Drawing for the job (mm, zero at the part's lowest x, y, z). Round coordinates to 2 decimals unless told otherwise and drop trailing zeros. Loops run counter-clockwise (first coordinate to the right, second up) from the corner with the lowest first, then second, coordinate; pieces in that order, holes last. Notation, with made-up numbers: (47, 3.5) - (86, 3.5) arc R10 ccw to (86, 8.5) - close; hole circle Ø1 at (-3, 57). An arc over 180 degrees is marked (long way). Put each result on its own line as item: value.
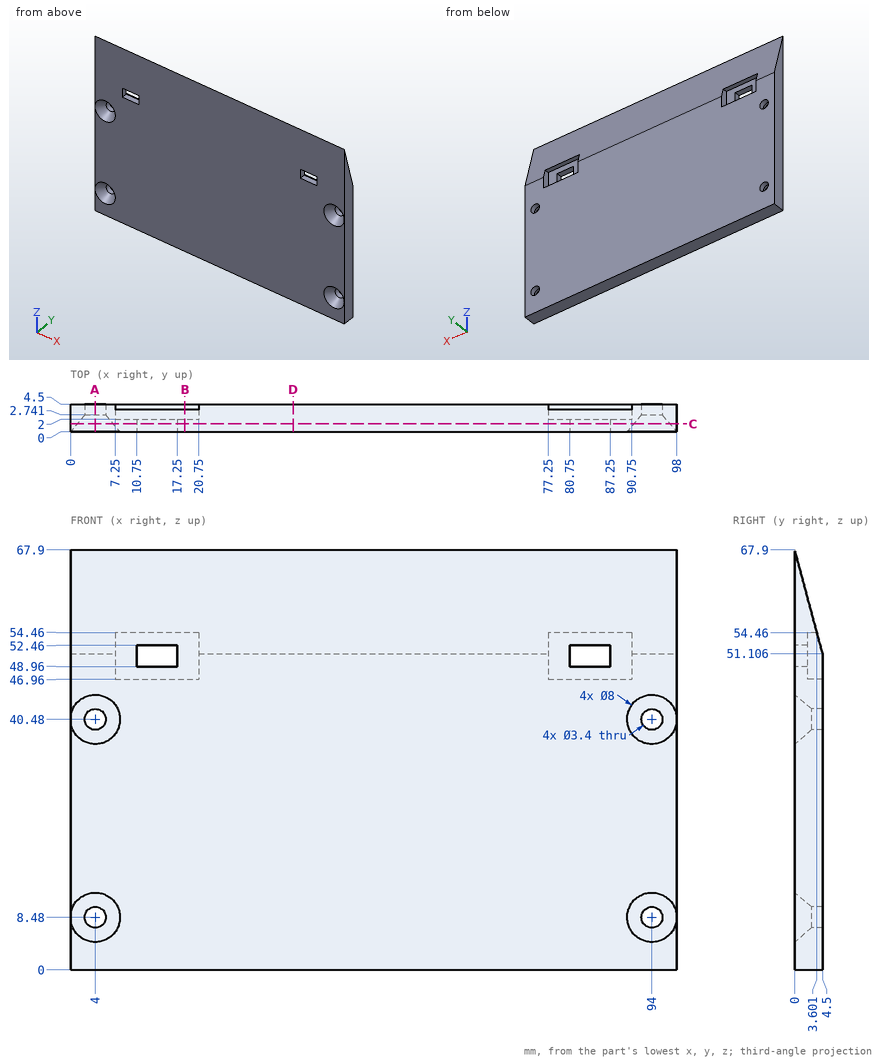
1. Band-saw the part on A-A (x = 4). List the corners of the cut face in (y, z).
A:
outline: (0, 0) - (4.5, 0) - (4.5, 6.78) - (2.74, 6.78) - (0, 4.48) - close; (0, 12.48) - (2.74, 10.18) - (4.5, 10.18) - (4.5, 38.78) - (2.74, 38.78) - (0, 36.48) - close; (0, 44.48) - (2.74, 42.18) - (4.5, 42.18) - (4.5, 51.11) - (0, 67.9) - close
2. Band-saw the part on B-B (x = 18.5). List the corners of the cut face in (y, z).
A:
outline: (0, 0) - (4.5, 0) - (4.5, 46.96) - (2, 46.96) - (2, 54.46) - (3.6, 54.46) - (0, 67.9) - close
3. Probe line 1 along X through (y, z) = (4, 8.48); line 2 along X through (y, z) = (3.15, 49); line 3 along Y through (x, z) = (47, 64.5). List the from-to ranges inside material, lowest first. Write a range as [from, to].
A:
line 1: x = [0, 2.3], [5.7, 92.3], [95.7, 98]
line 2: x = [0, 7.25], [20.75, 77.25], [90.75, 98]
line 3: y = [0, 0.91]
4. Band-saw the part on C-C (y = 1.3). List the corners of the cut face in (x, z).
A:
outline: (0, 0) - (98, 0) - (98, 63.05) - (0, 63.05) - close; hole circle Ø5.82 at (4, 8.48); hole circle Ø5.82 at (4, 40.48); hole (10.75, 48.96) - (17.25, 48.96) - (17.25, 52.46) - (10.75, 52.46) - close; hole (80.75, 48.96) - (87.25, 48.96) - (87.25, 52.46) - (80.75, 52.46) - close; hole circle Ø5.82 at (94, 8.48); hole circle Ø5.82 at (94, 40.48)
5. Band-saw the part on D-D (x = 36). List the corners of the cut face in (y, z), plus the area to 3 significant figures.
A:
outline: (0, 0) - (4.5, 0) - (4.5, 51.11) - (0, 67.9) - close
area: 268 mm²
